from build123d import *

# Parameters (mm, degrees)
SKETCH1_R            = 14.875
SKETCH1_R_2          = 11
BOSS_EXTRUDE13_DEPTH = 17
SKETCH1_14_R         = 24.34
SKETCH1_14_R_2       = 14.875
SKETCH1_14_R_3       = 2.5
BOSS_EXTRUDE14_DEPTH = 10
SKETCH1_16_R         = 11
SKETCH1_16_R_2       = 7.375
BOSS_EXTRUDE15_DEPTH = 1


with BuildPart() as part:
    # Sketch1 → Boss-Extrude13 (new body)
    with BuildSketch(Plane(origin=(0, 0, 0), x_dir=(1, 0, 0), z_dir=(0, 1, 0))):
        with Locations(Location((-14.907558872, 21.380040763, 0), (0, 0, 270))):
            Circle(SKETCH1_R)
        with Locations(Location((-14.907558872, 21.380040763, 0), (0, 0, 270))):
            Circle(SKETCH1_R_2, mode=Mode.SUBTRACT)
    extrude(amount=BOSS_EXTRUDE13_DEPTH)

    # Sketch1_14 → Boss-Extrude14 (add)
    with BuildSketch(Plane(origin=(0, 0, 0), x_dir=(1, 0, 0), z_dir=(0, 1, 0))):
        with Locations(Location((-14.907558872, 21.380040763, 0), (0, 0, 270))):
            Circle(SKETCH1_14_R)
        with Locations(Location((-14.907558872, 21.380040763, 0), (0, 0, 270))):
            Circle(SKETCH1_14_R_2, mode=Mode.SUBTRACT)
        with Locations(Location((0.098010813, 8.400885227, 0), (0, 0, 270))):
            Circle(SKETCH1_14_R_3, mode=Mode.SUBTRACT)
        with Locations(Location((-1.946083972, 36.400885227, 0), (0, 0, 270))):
            Circle(SKETCH1_14_R_3, mode=Mode.SUBTRACT)
        with Locations(Location((-27.824633533, 6.320997559, 0), (0, 0, 270))):
            Circle(SKETCH1_14_R_3, mode=Mode.SUBTRACT)
        with Locations(Location((-29.946083972, 34.320997559, 0), (0, 0, 270))):
            Circle(SKETCH1_14_R_3, mode=Mode.SUBTRACT)
    extrude(amount=BOSS_EXTRUDE14_DEPTH)

    # Sketch1_16 → Boss-Extrude15 (add)
    with BuildSketch(Plane(origin=(0, 0, 0), x_dir=(1, 0, 0), z_dir=(0, 1, 0))):
        with Locations(Location((-14.907558872, 21.380040763, 0), (0, 0, 270))):
            Circle(SKETCH1_16_R)
        with Locations(Location((-14.907558872, 21.380040763, 0), (0, 0, 270))):
            Circle(SKETCH1_16_R_2, mode=Mode.SUBTRACT)
    extrude(amount=BOSS_EXTRUDE15_DEPTH)


solid = part.part
Design review of the part built by this model. Coordinates are the model's own, in mm. A direction names the side the tool comes from. Give positions to 0.01 mm unless a question says otherwise; leave off trailing zeros. Loops run counter-clockwise (first coordinate to the right, second up) from the corner with the lowest first, then second, coordinate; pieces in that order, holes last. Notation, with made-up numbers: (-19, 14.25) - (-7, 14.25) arc R21 cw to (-7, 33.25) - close; hole circle Ø11 at (-39.75, 59.5). An arc over 180 degrees is marked (long way). Write item = value, one per line.
1) Clearance check with flat-ended pins moving along their axes: pin 1 Ø4 at (y, z) = (11.5, -5) entering from +X; pin 2 Ø13 at (x, z) = (-14.91, -21.38) entering from +Y; pin 3 Ø4 at (x, y) = (3, 6) entering from +Z; pin 4 Ø6.5 at (x, z) = (-1.95, -36.4) entering from +Y. State where each tip first meets the part, or that it passes through.
Result sheet:
pin_1 = 4.22
pin_2 = through
pin_3 = -2.96
pin_4 = 10
2) Draft analysis for pull direction Z (two halves, no side actions). For faces 1 (the face through (-2.365, 13.451, -13.383)), 2 (the face through (-15, 10, -5)), 3 (the face through (-21.6, 8.89, -30.11)), state which applies: +Z half, -Z half, draft (parallel to the pull), parting line (faces both ways), or undercut.
Result sheet:
face_1 = parting line
face_2 = draft
face_3 = undercut
3) Take a section at A-A on z = -20. State the section outline as (x, y) points, and give its area (3 significant figures).
Result sheet:
outline = (-39.21, 0) - (-22.15, 0) - (-22.15, 1) - (-25.82, 1) - (-25.82, 17) - (-29.72, 17) - (-29.72, 10) - (-39.21, 10) - close; (-7.66, 0) - (9.39, 0) - (9.39, 10) - (-0.1, 10) - (-0.1, 17) - (-3.99, 17) - (-3.99, 1) - (-7.66, 1) - close
area = 330 mm2
4) Take a section at D-D on z = -8. State the section outline as (x, y) points.
Result sheet:
outline = (-35.24, 0) - (-29.68, 0) - (-29.68, 10) - (-35.24, 10) - close; (-25.97, 0) - (-2.37, 0) - (-2.37, 10) - (-8.41, 10) - (-8.41, 17) - (-21.41, 17) - (-21.41, 10) - (-25.97, 10) - close; (2.57, 0) - (5.42, 0) - (5.42, 10) - (2.57, 10) - close
5) Take a section at B-B on x = -17. State the section outline as (y, z) points.
Result sheet:
outline = (0, -45.63) - (10, -45.63) - (10, -36.11) - (17, -36.11) - (17, -32.18) - (1, -32.18) - (1, -28.45) - (0, -28.45) - close; (0, -14.31) - (1, -14.31) - (1, -10.58) - (17, -10.58) - (17, -6.65) - (10, -6.65) - (10, 2.87) - (0, 2.87) - close
6) To check wall thickness, follow line 1 (Z direction, x = -14.5, y = 8.5); line 2 (Z direction, x = -14.5, y = 14); line 3 (X direction, y = 2, z = -36). State the ranges of each line that lie inside material, in increasing order.
Result sheet:
line_1 = -45.72 to -32.37, -10.39 to 2.96
line_2 = -36.25 to -32.37, -10.39 to -6.51
line_3 = -34.37 to -31.8, -28.09 to -4.41, 0.52 to 4.55
7) Take a section at C-C on y = 2.25. State the section outline as (x, z) points.
Result sheet:
outline = circle Ø48.68 at (-14.91, -21.38); hole circle Ø5 at (-29.95, -34.32); hole circle Ø5 at (-27.82, -6.32); hole circle Ø22 at (-14.91, -21.38); hole circle Ø5 at (-1.95, -36.4); hole circle Ø5 at (0.1, -8.4)
8) Tool access review of faces 4 (the face through (-29.718, 4.93, -40.695)), 5 (the face through (-17, 1, -14)): name each direction out of +Z, -Z, +X, -X, +Y, -Y from which nothing blocks a thin tool from reaching the whole face with its end or side.
Result sheet:
face_4 = +Y, -Y
face_5 = +Y
